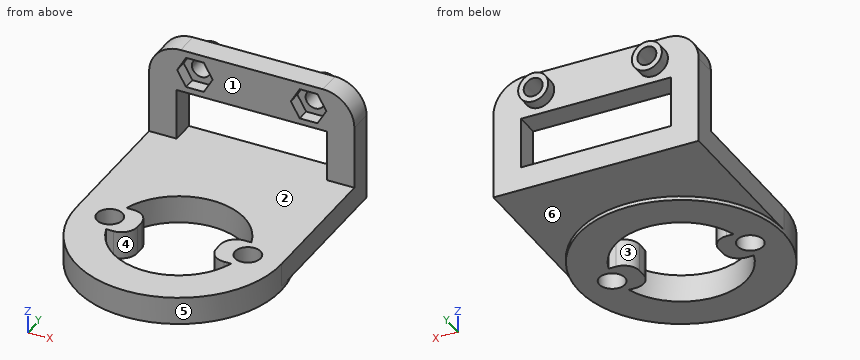
```python
from build123d import *

# Parameters (mm, degrees)
ESBO_O1_R                = 13
ESBO_O1_R_2              = 8.3
RESSALTO_EXTRUS_O1_DEPTH = 3.5
RESSALTO_EXTRUS_O2_DEPTH = 3.5
ESBO_O4_R                = 1.625
CORTE_EXTRUS_O2_DEPTH    = 19.714967272
FILETE1_R                = 2
RESSALTO_EXTRUS_O4_START = -3
RESSALTO_EXTRUS_O4_DEPTH = 3
RESSALTO_EXTRUS_O5_DEPTH = 3
ESBO_O9_R                = 1.9
RESSALTO_EXTRUS_O6_DEPTH = 1.5
ESBO_O10_R               = 1.2
CORTE_EXTRUS_O3_DEPTH    = 41.859515416
CORTE_EXTRUS_O4_DEPTH    = 1.6
FILETE2_R                = 4


with BuildPart() as part:
    # Esboço1 → Ressalto-extrusão1 (new body)
    with BuildSketch(Plane.XY):
        Circle(ESBO_O1_R)
        Circle(ESBO_O1_R_2, mode=Mode.SUBTRACT)
    extrude(amount=RESSALTO_EXTRUS_O1_DEPTH)

    # Esboço3 → Ressalto-extrusão2 (add, through all)
    with BuildSketch(Plane.XY.offset(3.5)):
        with BuildLine():
            Line((-8.124038405, 2.5), (-5, 2.5))
            Line((-5, 2.5), (-5, -2.5))
            Line((-5, -2.5), (-8.124038405, -2.5))
            ThreePointArc((-8.124038405, -2.5), (-8.5, 0), (-8.124038405, 2.5))
        make_face()
        with BuildLine():
            Line((5, 2.5), (5, -2.5))
            Line((5, -2.5), (8.124038405, -2.5))
            ThreePointArc((8.124038405, -2.5), (8.5, 0), (8.124038405, 2.5))
            Line((8.124038405, 2.5), (5, 2.5))
        make_face()
    extrude(amount=-RESSALTO_EXTRUS_O2_DEPTH)

    # Esboço4 → Corte-extrusão2 (cut, through all)
    with BuildSketch(Plane.XY.offset(3.5)):
        with Locations((-8.75, 0)):
            Circle(ESBO_O4_R)
        with Locations(Location((8.75, 0, 0), (0, 0, 180))):
            Circle(ESBO_O4_R)
    extrude(amount=-CORTE_EXTRUS_O2_DEPTH, mode=Mode.SUBTRACT)

    # Filete1
    filete1_edges = [part.edges().sort_by_distance(p)[0] for p in [
        (-5, 2.5, 1.75),
        (-5, -2.5, 1.75),
        (5, -2.5, 1.75),
        (5, 2.5, 1.75),
    ]]
    fillet(filete1_edges, radius=FILETE1_R)

    # Esboço7 → Ressalto-extrusão4 (add)
    with BuildSketch(Plane.XY.offset(3.5).offset(RESSALTO_EXTRUS_O4_START)):
        with BuildLine():
            Line((-13, 0), (-13, 21))
            Line((-13, 21), (13, 21))
            Line((13, 21), (13, 0))
            ThreePointArc((13, 0), (0, 13), (-13, 0))
        make_face()
    extrude(amount=RESSALTO_EXTRUS_O4_DEPTH)

    # Esboço8 → Ressalto-extrusão5 (add)
    with BuildSketch(Plane(origin=(0, 21, 0), x_dir=(1, 0, 0), z_dir=(0, 1, 0))):
        Polygon((-13, -3.5), (-13, -15.5), (13, -15.5), (13, -3.5), (9.5, -3.5), (9.5, -10), (-9.5, -10), (-9.5, -3.5), align=None)
    extrude(amount=-RESSALTO_EXTRUS_O5_DEPTH)

    # Esboço9 → Ressalto-extrusão6 (add)
    with BuildSketch(Plane(origin=(0, 21, 0), x_dir=(1, 0, 0), z_dir=(0, 1, 0))):
        with Locations(Location((-7.2, -12.7, 0), (0, 0, 270))):
            Circle(ESBO_O9_R)
        with Locations(Location((7.2, -12.7, 0), (0, 0, 90))):
            Circle(ESBO_O9_R)
    extrude(amount=RESSALTO_EXTRUS_O6_DEPTH)

    # Esboço10 → Corte-extrusão3 (cut, through all)
    with BuildSketch(Plane(origin=(0, 22.5, 0), x_dir=(1, 0, 0), z_dir=(0, 1, 0))):
        with Locations(Location((-7.2, -12.7, 0), (0, 0, 270))):
            Circle(ESBO_O10_R)
        with Locations(Location((7.2, -12.7, 0), (0, 0, 270))):
            Circle(ESBO_O10_R)
    extrude(amount=-CORTE_EXTRUS_O3_DEPTH, mode=Mode.SUBTRACT)

    # Esboço11 → Corte-extrusão4 (cut)
    with BuildSketch(Plane.XZ.offset(-18)):
        Polygon((-4.94833395, 12.7), (-6.074166975, 14.65), (-8.325833025, 14.65), (-9.45166605, 12.7), (-8.325833025, 10.75), (-6.074166975, 10.75), align=None)
        Polygon((6.074166975, 10.75), (4.94833395, 12.7), (6.074166975, 14.65), (8.325833025, 14.65), (9.45166605, 12.7), (8.325833025, 10.75), align=None)
    extrude(amount=-CORTE_EXTRUS_O4_DEPTH, mode=Mode.SUBTRACT)

    # Filete2
    filete2_edges = [part.edges().sort_by_distance(p)[0] for p in [
        (13, 19.5, 15.5),
        (-13, 19.5, 15.5),
    ]]
    fillet(filete2_edges, radius=FILETE2_R)


solid = part.part
```
Verification items for the finished model (mm, model axes). Face numbers are marked on the shaded views. A direction names the side the tool comes from. Coordinates: 2 decimals unless noted, no trailing zeros. Loops run counter-clockwise (first coordinate to the right, second up) from the corner with the lowest first, then second, coordinate; pieces in that order, holes last. Notation, with made-up numbers: (-13, 29) -> (-1, 29) arc R13 ccw to (-1, 46) -> close; hole circle Ø1 at (58, 82). An arc over 180 degrees is marked (long way). Answer in a Markdown table with one row per item. Add a question column.
1. Material ranges on probe 1 along X at (y, z) = (21.1, 12.7); probe 2 along Z at (x, y) = (6.5, 13); probe 3 along Z at (x, y) = (8.75, -9.5), recorded low to high. Write a range as [from, to].
2. Access from +Z, -Z, +X, -X, +Y, -Y to the whole of each face (thin tool, end or side, straight path). Record for the marked faces 4, 5 and 6.
3. Section check A-A, the plane z = 9. Enter the section's corners in (x, y), then the cut area to 3 significant figures.
4. Depth check by flat-ended pin: P1, Ø1, axis at x = -9, y = 14, coming from the -Z side; P2, Ø8, axis at x = 0.5, y = 15.5, coming from the -Z side; P3, Ø6, axis at x = 1.5, y = 10.5, coming from the +Z side; P4, Ø3, axis at x = -7.2, z = 12.7, coming from the -Y side. Enter the tip coordinate at first touch or a pass-through.
5. Section check D-D, the plane y = 1. Give the number of separate pieces and of enclosed holes in the cut face, then the cut area to 3 significant figures.
6. Section check C-C, the plane x = 0. Enter the section's corners in (y, z), then the cut area to 3 significant figures.
7. Section check B-B, the plane z = 1.75. Enter the section's corners in (x, y) (3 decimals).
8. Draft check along Y on the marked faces 1, 2 and 3. Enter one of: +Y half, -Y half, draft (parallel to the pull), parting line (faces both ways), or undercut.
Derived:
| question | item | result |
|---|---|---|
| 1 | probe 1 | x = [-9.1, -8.4], [-6, -5.3], [5.3, 6], [8.4, 9.1] |
| 1 | probe 2 | z = [0.5, 3.5] |
| 1 | probe 3 | z = [0, 3.5] |
| 2 | face 4 | +Z, -Z |
| 2 | face 5 | -Z |
| 2 | face 6 | -Z, +Y |
| 3 | outline | (-13, 18) -> (-9.5, 18) -> (-9.5, 21) -> (-13, 21) -> close; (9.5, 18) -> (13, 18) -> (13, 21) -> (9.5, 21) -> close |
| 3 | area | 21.0 mm² |
| 4 | P1 | stops at z = 0.5 |
| 4 | P2 | stops at z = 0 |
| 4 | P3 | stops at z = 3.5 |
| 4 | P4 | stops at y = 19.6 |
| 5 | separate pieces | 4 |
| 5 | enclosed holes | 0 |
| 5 | area | 37.6 mm² |
| 6 | outline | (-13, 0) -> (-8.3, 0) -> (-8.3, 3.5) -> (-13, 3.5) -> close; (8.3, 0) -> (13, 0) -> (13, 0.5) -> (21, 0.5) -> (21, 3.5) -> (8.3, 3.5) -> close; (18, 10) -> (21, 10) -> (21, 15.5) -> (18, 15.5) -> close |
| 6 | area | 73.4 mm² |
| 7 | outline | (-13, 0) arc R13 ccw to (13, 0) -> (13, 21) -> (-13, 21) -> close; hole circle Ø3.25 at (-8.75, 0); hole (-7.915, -2.5) arc R8.3 ccw to (7.915, -2.5) -> (7, -2.5) arc R2 cw to (5, -0.5) -> (5, 0.5) arc R2 cw to (7, 2.5) -> (7.915, 2.5) arc R8.3 ccw to (-7.915, 2.5) -> (-7, 2.5) arc R2 cw to (-5, 0.5) -> (-5, -0.5) arc R2 cw to (-7, -2.5) -> close; hole circle Ø3.25 at (8.75, 0) |
| 8 | face 1 | -Y half |
| 8 | face 2 | draft |
| 8 | face 3 | undercut |
